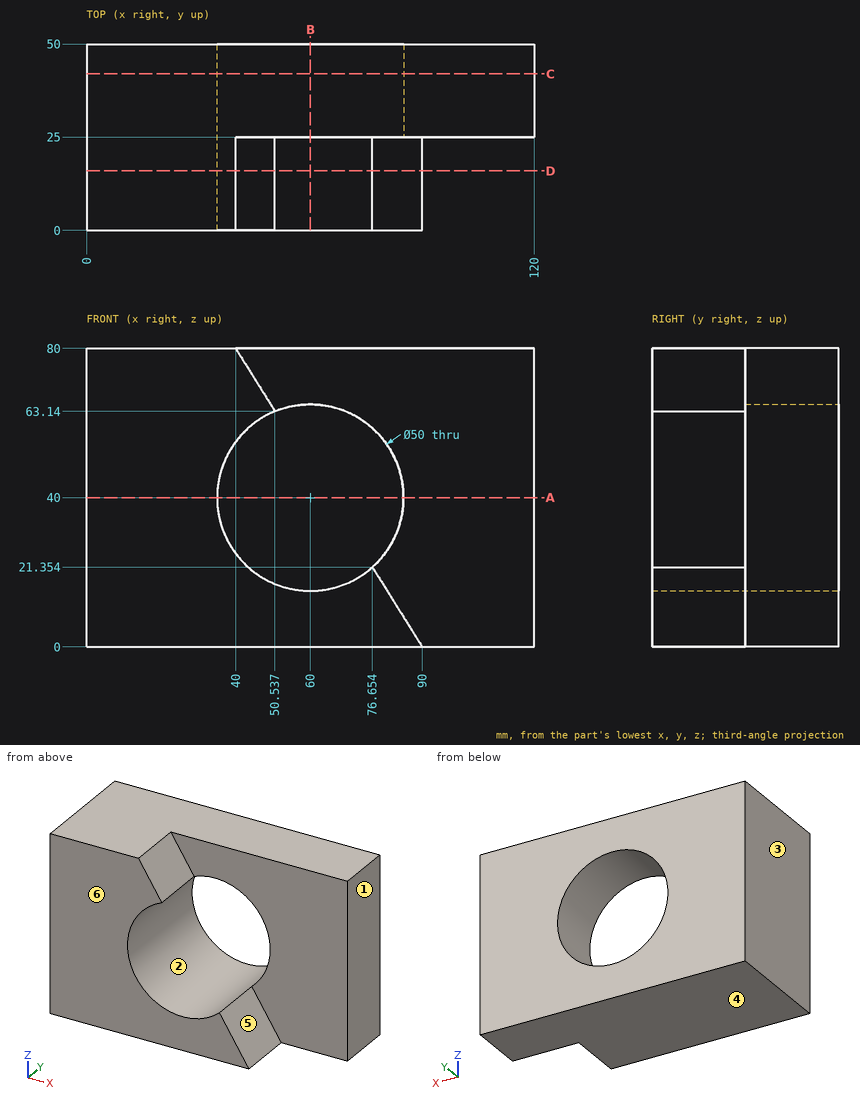
The figure shows three views and two pictorial views of one solid part (mm, origin at its lowest corner). Answer the questions. A direction names the side the tool comes from. Round coordinates to 2 decimals unless told otherwise and drop trailing zeros. Order: outer loops, then holes, each group sorted by start corner. A loop starts at its lowest first (then second) coordinate and runs counter-clockwise, first axis right, second up. Notation, with made-up numbers: (-38.75, 57.5) -> (-24.75, 57.5) arc R33 cw to (-24.75, 92.5) -> close; hole circle Ø5 at (44, 36.5). An arc over 180 degrees is marked (long way). Put each result on its own line as item: value.
Q1. Section B-B, the plane x = 60 is taken. Write down the section's boundary in (y, z), and give its area (4 significant figures).
Results list:
outline: (0, 0) -> (50, 0) -> (50, 15) -> (0, 15) -> close; (25, 65) -> (50, 65) -> (50, 80) -> (25, 80) -> close
area: 1,125 mm^2
Q2. Section A-A, the plane z = 40 is taken. Write down the section's boundary in (x, y).
Results list:
outline: (0, 0) -> (35, 0) -> (35, 50) -> (0, 50) -> close; (85, 25) -> (120, 25) -> (120, 50) -> (85, 50) -> close
Q3. Section D-D, the plane y = 16 is taken. Write down the section's boundary in (x, z) (1 decimal).
Results list:
outline: (0, 0) -> (90, 0) -> (76.7, 21.4) arc R25 cw (long way) to (50.5, 63.1) -> (40, 80) -> (0, 80) -> close
Q4. Section C-C, the plane y = 42 is taken. Write down the section's boundary in (x, z).
Results list:
outline: (0, 0) -> (120, 0) -> (120, 80) -> (0, 80) -> close; hole circle Ø50 at (60, 40)
Q5. Determine the mould class of the marked faces 1, 2, 3 and 4 for opening direction X: pulls with the +X half, pulls with the -X half, needs draft (parallel to the pull), parting line crosses it, or undercut.
Results list:
face 1: pulls with the +X half
face 2: undercut
face 3: pulls with the -X half
face 4: needs draft
Q6. This flat-tipped pin is pushed along its axis until it touches: P1, Ø6, axis at x = 58, z = 64.5, coming from the -Y side. Where does it stop, or does it pass through?
Results list:
P1: y = 25
Q7. Consider line 1 along Z through (x, y) = (60, 30); line 2 along Y through (x, z) = (91.5, 4.5); line 3 along Z through (x, y) = (60, 15.5). Determine where each line is inside the solid, lowest interval first.
Results list:
line 1: 0 to 15, 65 to 80
line 2: 25 to 50
line 3: 0 to 15
Q8. Which of the six approach directions +Z, -Z, +X, -X, +Y, -Y give full straight-line access (tool end or side, diameter ignored) to the marked faces 5 and 6?
Results list:
face 5: +Z, +X, -Y
face 6: +Z, -Z, +X, -X, -Y
